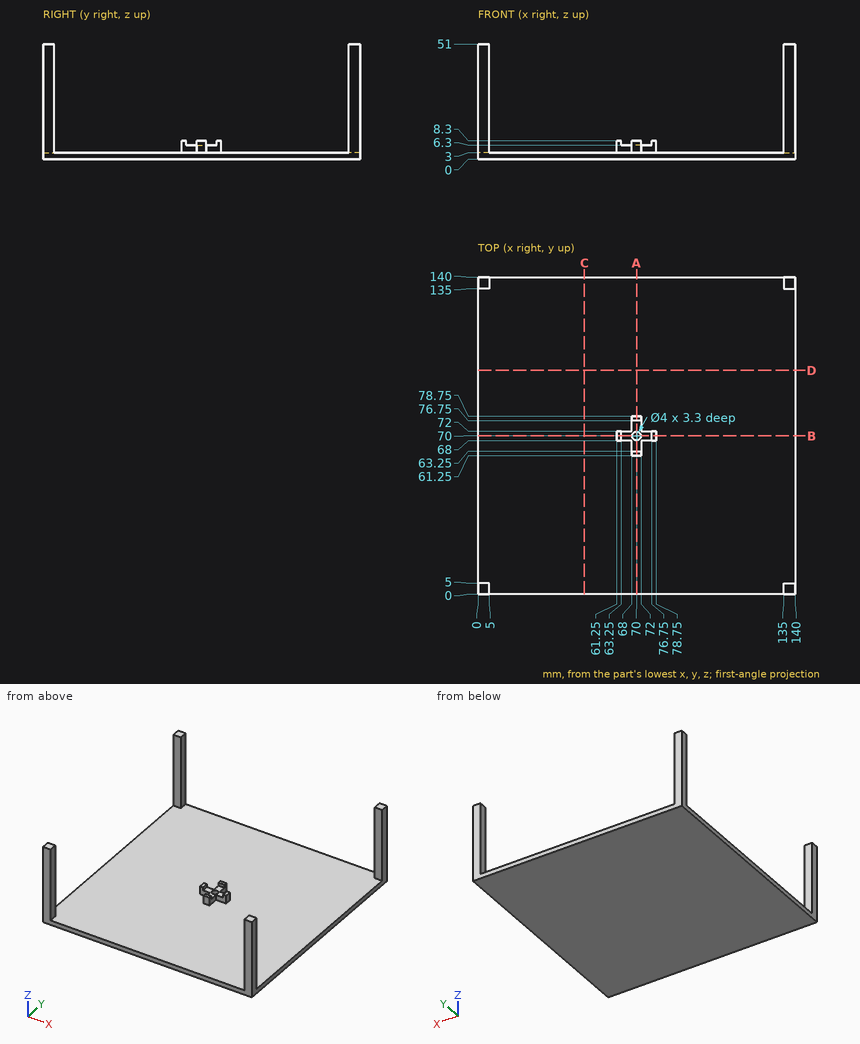
The drawing under review shows one solid part. Ordinate dimensions are in mm from its lowest x, y, z. Coordinates: 2 decimals unless noted, no trailing zeros. Loops run counter-clockwise (first coordinate to the right, second up) from the corner with the lowest first, then second, coordinate; pieces in that order, holes last. Notation, with made-up numbers: (72.25, 23) - (122.25, 23) arc R15 ccw to (122.25, 30) - close; hole circle Ø2 at (32.25, -36). An arc over 180 degrees is marked (long way). Use CSV: the item, a comma, the result in double quotes. Start each with the question number.
1. Clearance check with flat-ended pins moving along their axes: pin 1 (1.6 mm diameter, centred on x = 75.5, z = 6, fed in from -Y); pin 2 (2 mm diameter, centred on x = 77.5, y = 70.5, fed in from +Z); pin 3 (4 mm diameter, centred on x = 114, y = 83.5, fed in from -Z); pin 4 (3 mm diameter, centred on x = 34.5, y = 89.5, fed in from +Z). State where each tip first meets the part, or that it passes through.
2. To check wall thickness, follow probe 1 along Y at (x, z) = (70, 4.25); probe 2 along Z at (x, y) = (45.5, 34); probe 3 along Z at (x, y) = (71, 76). State the ranges of each line that lie inside material, in increasing order.
3. Add section C-C on x = 47. Give the boundary of the cut face in (y, z).
4. Add section A-A on x = 70. Give the boundary of the cut face in (y, z).
Resolved:
1,pin 1,"y = 68"
1,pin 2,"z = 8.3"
1,pin 3,"z = 0"
1,pin 4,"z = 3"
2,probe 1,"61.25 to 68, 72 to 78.75"
2,probe 2,"0 to 3"
2,probe 3,"0 to 6.3"
3,outline,"(0, 0) - (140, 0) - (140, 3) - (0, 3) - close"
4,outline,"(0, 0) - (140, 0) - (140, 3) - (78.75, 3) - (78.75, 8.3) - (76.75, 8.3) - (76.75, 6.3) - (72, 6.3) - (72, 3) - (68, 3) - (68, 6.3) - (63.25, 6.3) - (63.25, 8.3) - (61.25, 8.3) - (61.25, 3) - (0, 3) - close"
